Design review of the part built by this model. Coordinates are the model's own, in mm. Face numbers are marked on the shaded views. A direction names the side the tool comes from. Coordinates: 2 decimals unless noted, no trailing zeros. Write each loop counter-clockwise with the first axis right and the second up, starting at its lowest first coordinate (ties: lowest second). Pieces come first, ordered by that corner, then holes.
Q1. Take a section at A-A (z = 13.75). Give the boundary of the cut face in (x, y), and give its area (3 significant figures).
Q2. Insertion check: pin 1 (3 mm diameter, centred on x = 0, y = 0, fed in from -Z); pin 2 (8 mm diameter, centred on y = -5.5, z = 11, fed in from -X); pin 3 (5 mm diameter, centred on y = 5, z = 12, fed in from +X); pin 4 (5 mm diameter, centred on y = -3.5, z = 11, fed in from -X). Each pin has a flat end and moves straight along its axis. Give the tip position at first contact, or say it passes through.
Q3. Machinability: for the marked faces 4, 5 and 6, which of the approach directions +Z, -Z, +X, -X, +Y, -Y give a long, thin tool a straight path to every point of the face, cutting with its end or side? Answer none if there is none.
Q4. Take a section at B-B (z = 7.25). Give the boundary of the cut face in (x, y).
Q5. Mouldability with a two-part tool opening along Y and no side actions: class the marked faces 1, 2 and 3 as pulls with the +Y half, pulls with the -Y half, needs draft (parallel to the pull), parting line crosses it, or undercut.
Q6. For probe 1 along Y at (x, z) = (0, 15.5); probe 2 along X at (y, z) = (1.5, 4); probe 3 along X at (y, z) = (-2.25, 2.25), list the stretches that pass through material, from the lowest coordinate up.
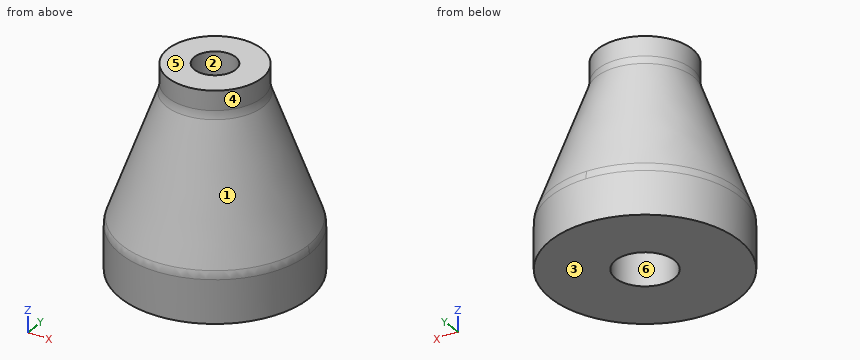
```python
from build123d import *

# Parameters (mm, degrees)
F0_R     = 8
F1_DEPTH = 17
F5_D     = 3.5
F7_D     = 5
F7_DEPTH = 10
F7_TIP   = 1.5021515476
F8_R     = 2


with BuildPart() as f1:
    # F0 (on Top) → F1 (new body)
    with BuildSketch(Plane.XY):
        Circle(F0_R)
    extrude(amount=F1_DEPTH)

    # F2 (on Right) → F3 (revolve, cut)
    with BuildSketch(Plane.YZ):
        Polygon((4, 15), (8, 4), (8, 17), (4, 17), align=None)
    revolve(axis=Axis((0, 0, 9.1980583966), (0, 0, 1)), mode=Mode.SUBTRACT)

    # F5 (through all)
    with Locations(Plane.XY.offset(17)):
        with Locations((0, 0)):
            Hole(F5_D / 2)

    # F7
    with Locations(Plane(origin=(0, 0, 0), x_dir=(1, 0, 0), z_dir=(0, 0, -1))):
        with Locations((0, 0)):
            Hole(F7_D / 2, depth=F7_DEPTH)
            with Locations((0, 0, -(F7_DEPTH + F7_TIP / 2))):  # 118° drill point
                Cone(0, F7_D / 2, F7_TIP, mode=Mode.SUBTRACT)

    # F8
    f8_edges = [f1.edges().sort_by_distance(p)[0] for p in [
        (0, 6, 9.5),
        (-5.656854, -5.656854, 4),
        (5.656854, 5.656854, 4),
        (0, -4, 15),
    ]]
    fillet(f8_edges, radius=F8_R)


solid = f1.part
```
Response:
1. outline: circle Ø8.91 at (0, 0); hole circle Ø3.5 at (0, 0)
1. area: 52.7 mm2
2. pin 1: passes through
2. pin 2: stops at x = -5.91
2. pin 3: stops at x = 4.77
2. pin 4: stops at x = -5.85
3. face 4: +Z
3. face 5: +Z, +X, -X, +Y, -Y
3. face 6: -Z
4. outline: circle Ø13.64 at (0, 0); hole circle Ø5 at (0, 0)
5. face 1: parting line crosses it
5. face 2: undercut
5. face 3: needs draft
6. probe 1: y = -4 to -1.75, 1.75 to 4
6. probe 2: x = -7.83 to -2, 2 to 7.83
6. probe 3: x = -7.68 to -1.09, 1.09 to 7.68
